Can you work these out from the model? Positions are in its coordinate system, mm. A direction names the side the tool comes from. Round coordinates to 2 decimals unless told otherwise and drop trailing zeros. Loops run counter-clockwise (first coordinate to the right, second up) from the corner with the lowest first, then second, coordinate; pieces in that order, holes last.
(1) If I drill on line 1 along Z through (x, y) = (5.25, 0.4); line 2 along Y through (x, z) = (5, 1.5); line 3 along Z through (x, y) = (8, 3.15), over which ranges is the centre line in solid material (lowest first)?
(2) I want a section at C-C on y = 3.65. Write out the boundary of the cut face in (x, z).
(3) I want a section at B-B on y = 2. Write out the boundary of the cut face in (x, z), plus the area to 3 significant figures.
(4) Will this pin go through, and if not, where does the flat tip stop? pin 1 Ø2 at (y, z) = (3, 6) entering from +X.
(5) I want a section at A-A on z = 5. Write out the boundary of the cut face in (x, y).
(6) Thinking about a two-plate mould opening in Z: for faces 1 (the face through (5.3, 4, 0.4)), 2 (the face through (7.126, 2.276, 8.189)), 3 (the face through (8.95, 2, 5)), 4 (the face through (5, 2, 0)), which applies, released by +Z, released by -Z, zero draft, split by the parting line, or undercut?
(7) Which directions (+Z, -Z, +X, -X, +Y, -Y) give clear straight access to the entire face, cutting with the end or side of a thin tool? Please do faces 5 (the face through (3.43, 2.28, 8.22)), 6 (the face through (9.5, 2.4, 4.9)).
(8) I want a section at D-D on x = 6. Write out the boundary of the cut face in (y, z).
from build123d import *

# Parameters (mm, degrees)
F1_DEPTH = 10
F3_START = -0.6
F2_R     = 2.25
F3_DEPTH = 3.401
F4_DEPTH = 0.6


with BuildPart() as f1:
    # F0 (on Top) → F1 (new body)
    with BuildSketch(Plane.XY):
        Polygon((0, 1.4), (0, 0), (10.5, 0), (10.5, 1.4), (7.9, 4), (2.6, 4), align=None)
    extrude(amount=F1_DEPTH)

    # F2 (on face) → F3 (cut)
    with BuildSketch(Plane.XZ.offset(F3_START)):
        Polygon((8.95, 2.863804004), (8.95, 7.136195996), (5.25, 9.272391992), (1.55, 7.136195996), (1.55, 2.863804004), (5.25, 0.727608008), align=None)
        with Locations((5.25, 5)):
            Circle(F2_R, mode=Mode.SUBTRACT)
        with Locations((5.25, 5)):
            Circle(F2_R)
    extrude(amount=-F3_DEPTH, mode=Mode.SUBTRACT)

    # F2 (on face) → F4 (cut, through all)
    with BuildSketch(Plane.XZ):
        with Locations((5.25, 5)):
            Circle(F2_R)
    extrude(amount=-F4_DEPTH, mode=Mode.SUBTRACT)


solid = f1.part
Filled sheet:
1. line 1: z = 0 to 2.75, 7.25 to 10
1. line 2: y = 0 to 0.6
1. line 3: z = 0 to 2.32, 7.68 to 10
2. outline: (2.25, 0) - (8.25, 0) - (8.25, 2.46) - (5.25, 0.73) - (2.25, 2.46) - close; (2.25, 7.54) - (5.25, 9.27) - (8.25, 7.54) - (8.25, 10) - (2.25, 10) - close
3. outline: (0.6, 0) - (9.9, 0) - (9.9, 10) - (0.6, 10) - close; hole (1.55, 2.86) - (5.25, 0.73) - (8.95, 2.86) - (8.95, 7.14) - (5.25, 9.27) - (1.55, 7.14) - close
3. area: 45.6 mm2
4. pin 1: stops at x = 9.9
5. outline: (0, 0) - (3, 0) - (3, 0.6) - (1.55, 0.6) - (1.55, 2.95) - (0, 1.4) - close; (7.5, 0) - (10.5, 0) - (10.5, 1.4) - (8.95, 2.95) - (8.95, 0.6) - (7.5, 0.6) - close
6. face 1: zero draft
6. face 2: undercut
6. face 3: undercut
6. face 4: released by -Z
7. face 5: +Y
7. face 6: +Z, -Z, +X, +Y
8. outline: (0, 0) - (4, 0) - (4, 1.16) - (0.6, 1.16) - (0.6, 2.88) - (0, 2.88) - close; (0, 7.12) - (0.6, 7.12) - (0.6, 8.84) - (4, 8.84) - (4, 10) - (0, 10) - close
